```python
from build123d import *

# Parameters (mm, degrees)
SKETCH1_W           = 50.8
SKETCH1_H           = 50.8
BOSS_EXTRUDE1_DEPTH = 3.175
SKETCH2_R           = 14.35
CUT_EXTRUDE1_DEPTH  = 3.175
CUT_EXTRUDE2_DEPTH  = 3.175


with BuildPart() as part:
    # Sketch1 → Boss-Extrude1 (new body)
    with BuildSketch(Plane(origin=(0, 0, 0), x_dir=(1, 0, 0), z_dir=(0, 1, 0))):
        Rectangle(SKETCH1_W, SKETCH1_H)
    extrude(amount=BOSS_EXTRUDE1_DEPTH)

    # Sketch2 → Cut-Extrude1 (cut)
    with BuildSketch(Plane(origin=(0, 3.175, 0), x_dir=(1, 0, 0), z_dir=(0, 1, 0))):
        Circle(SKETCH2_R)
    extrude(amount=-CUT_EXTRUDE1_DEPTH, mode=Mode.SUBTRACT)

    # Sketch3 → Cut-Extrude2 (cut)
    with BuildSketch(Plane(origin=(0, 3.175, 0), x_dir=(1, 0, 0), z_dir=(0, 1, 0))):
        Polygon((-25.4, 25.4), (-24.638, 25.4), (-25.4, 24.638), align=None)
        Polygon((25.4, 25.4), (25.4, 24.638), (24.638, 25.4), align=None)
    extrude(amount=-CUT_EXTRUDE2_DEPTH, mode=Mode.SUBTRACT)


solid = part.part
```
Here's how the part is built. I have some questions about the finished solid (model axes, mm). Give positions to 0.01 mm unless a question says otherwise; leave off trailing zeros. Order: outer loops, then holes, each group sorted by start corner. A loop starts at its lowest first (then second) coordinate and runs counter-clockwise, first axis right, second up. Notation, with made-up numbers: (-18.5, 73.25) -> (40.5, 73.25) arc R15 ccw to (40.5, 90.25) -> close; hole circle Ø1 at (71.25, 20.25). An arc over 180 degrees is marked (long way). Use CSV: the item, a comma, the result in double quotes. Start each with the question number.
Item 1: Suppose I cut it at A-A (y = 1.35). List the corners of the cut face in (x, z) for me.
Item 2: Thinking about a two-plate mould opening in Z: for faces 1 (the cylindrical face through (7.714, 1.61, -12.1)), 2 (the flat face through (0, 2, 25.4)), 3 (the flat face through (-25.4, 2, 1)), which applies, pulls with the +Z half, pulls with the -Z half, needs draft (parallel to the pull), parting line crosses it, or undercut?
Item 3: If I drill on probe 1 along Z at (x, y) = (0, 0.85); probe 2 along X at (y, z) = (1.8, -12), over which ranges is the centre line in solid material (lowest first)? Write a range as [from, to].
Item 4: Suppose I cut it at C-C (x = 0). List the corners of the cut face in (y, z) for me (3 decimals).
Item 5: Suppose I cut it at B-B (z = 0). List the corners of the cut face in (x, y) for me (3 decimals).
Answer block:
1,outline,"(-25.4, -24.64) -> (-24.64, -25.4) -> (24.64, -25.4) -> (25.4, -24.64) -> (25.4, 25.4) -> (-25.4, 25.4) -> close; hole circle Ø28.7 at (0, 0)"
2,face 1,"undercut"
2,face 2,"pulls with the +Z half"
2,face 3,"needs draft"
3,probe 1,"z = [-25.4, -14.35], [14.35, 25.4]"
3,probe 2,"x = [-25.4, -7.87], [7.87, 25.4]"
4,outline,"(0, -25.4) -> (3.175, -25.4) -> (3.175, -14.35) -> (0, -14.35) -> close; (0, 14.35) -> (3.175, 14.35) -> (3.175, 25.4) -> (0, 25.4) -> close"
5,outline,"(-25.4, 0) -> (-14.35, 0) -> (-14.35, 3.175) -> (-25.4, 3.175) -> close; (14.35, 0) -> (25.4, 0) -> (25.4, 3.175) -> (14.35, 3.175) -> close"
